from build123d import *

# Parameters (mm, degrees)
F1_DEPTH  = 25.4
F2_R      = 6.35
F3_DEPTH  = 50.801
F5_DEPTH  = 50.801
F6_R      = 6.35
F7_DEPTH  = 12.701
F9_DEPTH  = 12.701
F11_DEPTH = 12.701


with BuildPart() as f1:
    # F0 (on Front) → F1 (new body)
    with BuildSketch(Plane.XZ):
        Polygon((-51.843755758, 12.7), (-51.843755758, 0), (24.356244242, 0), (24.356244242, 12.7), (-1.043755758, 12.7), (-1.043755758, 44.45), (-26.443755758, 44.45), (-26.443755758, 12.7), align=None)
    extrude(amount=F1_DEPTH)

    # F2 (on face) → F3 (cut, through all)
    with BuildSketch(Plane(origin=(-26.443755758, 0, 0), x_dir=(0, -1, 0), z_dir=(-1, 0, 0))):
        with Locations((12.7, 31.75)):
            Circle(F2_R)
    extrude(amount=-F3_DEPTH, mode=Mode.SUBTRACT)

    # F4 (on face) → F5 (cut, through all)
    with BuildSketch(Plane.YZ.offset(-1.043755758)):
        with BuildLine():
            ThreePointArc((-25.4, 38.1), (-12.6975472927, 44.4155540641), (0, 38.0901433527))
            Line((0, 38.0901433527), (0, 44.45))
            Line((0, 44.45), (-25.4, 44.45))
            Line((-25.4, 44.45), (-25.4, 38.1))
        make_face()
    extrude(amount=-F5_DEPTH, mode=Mode.SUBTRACT)

    # F6 (on face) → F7 (cut, through all)
    with BuildSketch(Plane.XY.offset(12.7)):
        with Locations((-39.143755758, -12.7)):
            Circle(F6_R)
        with Locations((11.656244242, -12.7)):
            Circle(F6_R)
    extrude(amount=-F7_DEPTH, mode=Mode.SUBTRACT)

    # F8 (on face) → F9 (cut, through all)
    with BuildSketch(Plane.XY.offset(12.7)):
        with BuildLine():
            ThreePointArc((-45.493755758, -25.4), (-49.7807083247, -20.6909850484), (-51.843755758, -14.6663174715))
            Line((-51.843755758, -14.6663174715), (-51.843755758, -25.4))
            Line((-51.843755758, -25.4), (-45.493755758, -25.4))
        make_face()
        with BuildLine():
            ThreePointArc((-51.843755758, -10.7336825285), (-49.7807083247, -4.7090149516), (-45.493755758, 0))
            Line((-45.493755758, 0), (-51.843755758, 0))
            Line((-51.843755758, 0), (-51.843755758, -10.7336825285))
        make_face()
    extrude(amount=-F9_DEPTH, mode=Mode.SUBTRACT)

    # F10 (on face) → F11 (cut, through all)
    with BuildSketch(Plane.XY.offset(12.7)):
        with BuildLine():
            ThreePointArc((18.006244242, 0), (24.3479033898, -12.7), (18.006244242, -25.4))
            Line((18.006244242, -25.4), (24.356244242, -25.4))
            Line((24.356244242, -25.4), (24.356244242, 0))
            Line((24.356244242, 0), (18.006244242, 0))
        make_face()
    extrude(amount=-F11_DEPTH, mode=Mode.SUBTRACT)


solid = f1.part
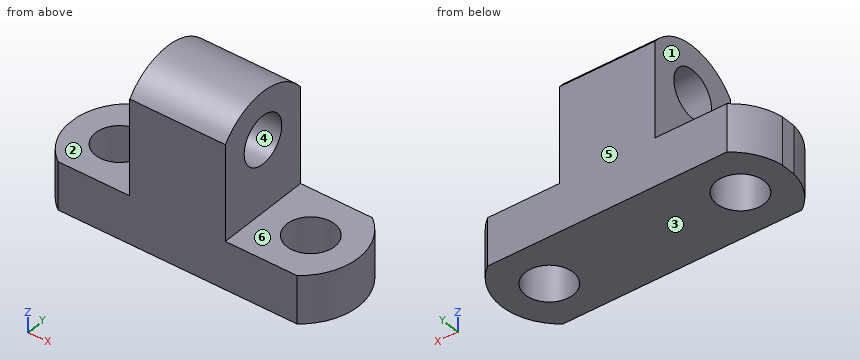
Build history of the part. All positions in model axes, mm. Face numbers are marked on the shaded views. A direction names the side the tool comes from. Coordinates: 2 decimals unless noted, no trailing zeros. Write each loop counter-clockwise with the first axis right and the second up, starting at its lowest first coordinate (ties: lowest second). Pieces come first, ordered by that corner, then holes. Notation, with made-up numbers: (6, -16.75) -> (34, -16.75) arc R36 ccw to (34, 18.25) -> close; hole circle Ø6 at (86, 71.25). An arc over 180 degrees is marked (long way). Use CSV: the item, a comma, the result in double quotes. Start each with the question number.
Q1. 3-axis set-ups, long thin cutter, end or side, ignore diameter. For the marked faces 5 and 6: which of +Z, -Z, +X, -X, +Y, -Y reach the whole face in a straight line?
Q2. Cut at A-A, the plane z = 9. List the corners of the cut face in (x, y), then the cut area to 3 significant figures.
Q3. Pull direction Z, two halves, no side cores. Call the marked faces 1, 2, 3 and 4: released by +Z, released by -Z, zero draft, split by the parting line, or undercut.
Q4. Cut at D-D, the plane z = 31.75. List the corners of the cut face in (x, y).
Q5. Cut at B-B, the plane y = -12.7. List the corners of the cut face in (x, z), then the cut area to 3 significant figures.
Q6. Drill centre lines: probe 1 along Z at (x, y) = (-39, -23); probe 2 along Z at (x, y) = (-3, -9.5); probe 3 along Z at (x, y) = (-21, -11.5). Where is each one in solid material? Low to high.
Q7. Flat gauge pins, fed straight in: pin 1 Ø7.5 at (y, z) = (-12, 31.5) entering from +X; pin 2 Ø12.5 at (x, y) = (-40.5, -10) entering from +Z; pin 3 Ø14.5 at (y, z) = (-12.7, 31.75) entering from -X; pin 4 Ø6 at (x, y) = (-15, -17) entering from -Z. Where does each tip first touch, or does it go through?
Q8. Cut at C-C, the plane x = 14.5. List the corners of the cut face in (y, z).
Checked values:
1,face 5,"+Z, -Z, +X, -X, +Y"
1,face 6,"+Z, +X, +Y, -Y"
2,outline,"(-51.84, -14.67) arc R15.69 ccw to (-45.49, -25.4) -> (18.01, -25.4) arc R15.89 ccw to (18.01, 0) -> (-45.49, 0) arc R15.69 ccw to (-51.84, -10.73) -> close; hole circle Ø12.7 at (-39.14, -12.7); hole circle Ø12.7 at (11.66, -12.7)"
2,area,"1,590 mm²"
3,face 1,"zero draft"
3,face 2,"released by +Z"
3,face 3,"released by -Z"
3,face 4,"undercut"
4,outline,"(-26.44, -25.4) -> (-1.04, -25.4) -> (-1.04, -19.05) -> (-26.44, -19.05) -> close; (-26.44, -6.35) -> (-1.04, -6.35) -> (-1.04, 0) -> (-26.44, 0) -> close"
5,outline,"(-51.84, 0) -> (-45.49, 0) -> (-45.49, 12.7) -> (-51.84, 12.7) -> close; (-32.79, 0) -> (5.31, 0) -> (5.31, 12.7) -> (-1.04, 12.7) -> (-1.04, 25.4) -> (-26.44, 25.4) -> (-26.44, 12.7) -> (-32.79, 12.7) -> close; (-26.44, 38.1) -> (-1.04, 38.1) -> (-1.04, 44.42) -> (-26.44, 44.42) -> close; (18.01, 0) -> (24.35, 0) -> (24.35, 12.7) -> (18.01, 12.7) -> close"
5,area,"1,130 mm²"
6,probe 1,"z = 0 to 12.7"
6,probe 2,"z = 0 to 26.27, 37.23 to 44.09"
6,probe 3,"z = 0 to 25.51, 37.99 to 44.37"
7,pin 1,"passes through"
7,pin 2,"stops at z = 12.7"
7,pin 3,"stops at x = -26.44"
7,pin 4,"stops at z = 0"
8,outline,"(-25.4, 0) -> (-18.38, 0) -> (-18.38, 12.7) -> (-25.4, 12.7) -> close; (-7.02, 0) -> (0, 0) -> (0, 12.7) -> (-7.02, 12.7) -> close"
